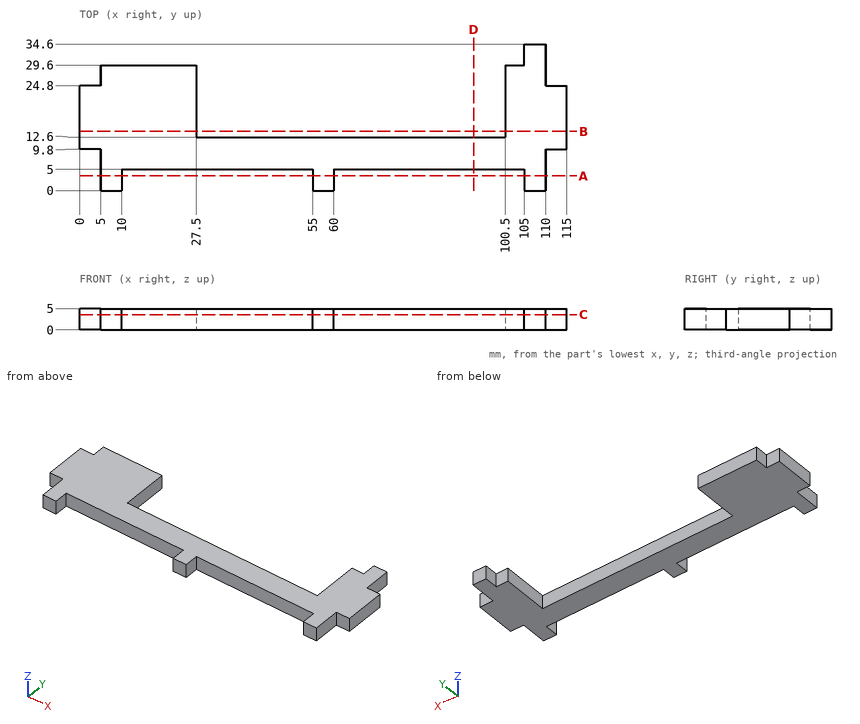
Here's the drawing with two shaded views (mm, measured from the low corner). I have some questions. Round coordinates to 2 decimals unless told otherwise and drop trailing zeros. Loops run counter-clockwise (first coordinate to the right, second up) from the corner with the lowest first, then second, coordinate; pieces in that order, holes last. Notation, with made-up numbers: (6.5, 41) - (22.5, 41) arc R30 cw to (22.5, 72) - close; hole circle Ø2 at (30.5, 89.25). An arc over 180 degrees is marked (long way). Use CSV: the item, a comma, the result in double quotes. Start each with the question number.
1) For pin 1 Ø2.5 at (y, z) = (7, 2) entering from +X; pin 2 Ø2.5 at (x, z) = (111.5, 1.5) entering from -Y; pin 3 Ø1.5 at (x, z) = (91, 2) entering from -Y, each with a flat end and sliding along its axis, tell me the tip position at first contact or that it passes through.
2) If we section it at A-A on y = 3.5: Write out the boundary of the cut face in (x, z), plus the area to 3 significant figures.
3) If we section it at B-B on y = 14: Write out the boundary of the cut face in (x, z).
4) If we section it at C-C on z = 3.6: Write out the boundary of the cut face in (x, y).
5) Please list where these lines run through material, in increasing order: probe 1 along X at (y, z) = (3, 3.3); probe 2 along X at (y, z) = (24.5, 4.6); probe 3 along X at (y, z) = (26, 0.4). Write a range as [from, to].
6) If we section it at D-D on x = 93: Write out the boundary of the cut face in (y, z), plus the area to 3 significant figures.
Geometry results:
1,pin 1,"stops at x = 110"
1,pin 2,"stops at y = 9.8"
1,pin 3,"stops at y = 5"
2,outline,"(5, 0) - (10, 0) - (10, 5) - (5, 5) - close; (55, 0) - (60, 0) - (60, 5) - (55, 5) - close; (105, 0) - (110, 0) - (110, 5) - (105, 5) - close"
2,area,"75.0 mm2"
3,outline,"(0, 0) - (27.5, 0) - (27.5, 5) - (0, 5) - close; (100.5, 0) - (115, 0) - (115, 5) - (100.5, 5) - close"
4,outline,"(0, 9.8) - (5, 9.8) - (5, 0) - (10, 0) - (10, 5) - (55, 5) - (55, 0) - (60, 0) - (60, 5) - (105, 5) - (105, 0) - (110, 0) - (110, 9.8) - (115, 9.8) - (115, 24.8) - (110, 24.8) - (110, 34.6) - (105, 34.6) - (105, 29.6) - (100.5, 29.6) - (100.5, 12.6) - (27.5, 12.6) - (27.5, 29.6) - (5, 29.6) - (5, 24.8) - (0, 24.8) - close"
5,probe 1,"x = [5, 10], [55, 60], [105, 110]"
5,probe 2,"x = [0, 27.5], [100.5, 115]"
5,probe 3,"x = [5, 27.5], [100.5, 110]"
6,outline,"(5, 0) - (12.6, 0) - (12.6, 5) - (5, 5) - close"
6,area,"38.0 mm2"
